Source: CAD feature listing. Evaluate the final solid. Frame: model axes, mm. A direction names the side the tool comes from. Give positions to 0.01 mm unless a question says otherwise; leave off trailing zeros. Loops run counter-clockwise (first coordinate to the right, second up) from the corner with the lowest first, then second, coordinate; pieces in that order, holes last. Notation, with made-up numbers: (-6, 77.25) - (1, 77.25) arc R26 cw to (1, 102.25) - close; hole circle Ø6 at (34.5, -2.75). An arc over 180 degrees is marked (long way). Put each result on its own line as item: value.
```python
from build123d import *

# Parameters (mm, degrees)
MODEL_R                 = 1.5
SALIENTE_EXTRUIR1_DEPTH = 3


with BuildPart() as part:
    # Model → Saliente-Extruir1 (new body)
    with BuildSketch(Plane.XY):
        with BuildLine():
            Line((256.429131311, 228.742243614), (346.429131311, 228.742243614))
            ThreePointArc((346.429131311, 228.742243614), (349.611111826, 227.424224129), (350.929131311, 224.242243614))
            Line((350.929131311, 224.242243614), (350.929131311, 215.242243614))
            ThreePointArc((350.929131311, 215.242243614), (349.611111826, 212.060263099), (346.429131311, 210.742243614))
            Line((346.429131311, 210.742243614), (256.429131311, 210.742243614))
            ThreePointArc((256.429131311, 210.742243614), (253.247150795, 212.060263099), (251.929131311, 215.242243614))
            Line((251.929131311, 215.242243614), (251.929131311, 224.242243614))
            ThreePointArc((251.929131311, 224.242243614), (253.247150795, 227.424224129), (256.429131311, 228.742243614))
        make_face()
        with Locations((337.429131311, 215.242243614)):
            Circle(MODEL_R, mode=Mode.SUBTRACT)
        with Locations((319.429131311, 215.242243614)):
            Circle(MODEL_R, mode=Mode.SUBTRACT)
        with Locations((328.429131311, 215.242243614)):
            Circle(MODEL_R, mode=Mode.SUBTRACT)
        with Locations((310.429131311, 215.242243614)):
            Circle(MODEL_R, mode=Mode.SUBTRACT)
        with Locations((292.429131311, 215.242243614)):
            Circle(MODEL_R, mode=Mode.SUBTRACT)
        with Locations((301.429131311, 215.242243614)):
            Circle(MODEL_R, mode=Mode.SUBTRACT)
        with Locations((274.429131311, 215.242243614)):
            Circle(MODEL_R, mode=Mode.SUBTRACT)
        with Locations((283.429131311, 215.242243614)):
            Circle(MODEL_R, mode=Mode.SUBTRACT)
        with Locations((265.429131311, 215.242243614)):
            Circle(MODEL_R, mode=Mode.SUBTRACT)
        with Locations((256.429131311, 215.242243614)):
            Circle(MODEL_R, mode=Mode.SUBTRACT)
        with Locations((346.429131311, 215.242243614)):
            Circle(MODEL_R, mode=Mode.SUBTRACT)
        with BuildLine():
            Line((256.429131311, 225.742243614), (346.429131311, 225.742243614))
            ThreePointArc((346.429131311, 225.742243614), (347.929131311, 224.242243614), (346.429131311, 222.742243614))
            Line((346.429131311, 222.742243614), (256.429131311, 222.742243614))
            ThreePointArc((256.429131311, 222.742243614), (254.929131311, 224.242243614), (256.429131311, 225.742243614))
        make_face(mode=Mode.SUBTRACT)
    extrude(amount=SALIENTE_EXTRUIR1_DEPTH)


solid = part.part
```
1) Section query A-A, the plane x = 297.5. Output: boundary loops of the cut face in (y, z).
Check result:
outline: (210.74, 0) - (222.74, 0) - (222.74, 3) - (210.74, 3) - close; (225.74, 0) - (228.74, 0) - (228.74, 3) - (225.74, 3) - close
2) Section query D-D, the plane y = 212.5. Output: boundary loops of the cut face in (x, z), plus the area to 3 significant figures.
Check result:
outline: (252.86, 0) - (350, 0) - (350, 3) - (252.86, 3) - close
area: 291 mm²
3) Material intervals for line 1 along Y through (x, z) = (301.5, 0.3); line 2 along Y through (x, z) = (282.5, 0.95); line 3 along Y through (x, z) = (278, 2.85), sorted ascending. Write a range as [from, to].
Check result:
line 1: [210.74, 213.74], [216.74, 222.74], [225.74, 228.74]
line 2: [210.74, 214.06], [216.42, 222.74], [225.74, 228.74]
line 3: [210.74, 222.74], [225.74, 228.74]
4) Mould query, pull axis Y, two halves, no side actions, for faces 1 (the flat face through (302, 220, 0)), 2 (the flat face through (301, 228.742, 1)), 3 (the cylindrical face through (300.324, 216.256, 1.479)). Classes: pulls with the +Y half, pulls with the -Y half, needs draft (parallel to the pull), parting line crosses it, or undercut.
Check result:
face 1: needs draft
face 2: pulls with the +Y half
face 3: undercut
5) Section query C-C, the plane x = 265.5. Output: boundary loops of the cut face in (y, z).
Check result:
outline: (210.74, 0) - (213.74, 0) - (213.74, 3) - (210.74, 3) - close; (216.74, 0) - (222.74, 0) - (222.74, 3) - (216.74, 3) - close; (225.74, 0) - (228.74, 0) - (228.74, 3) - (225.74, 3) - close
6) Access query for faces 4 (the flat face through (302, 210.742, 1)), 5 (the cylindrical face through (347.93, 224.28, 1.48)). Directions: +Z, -Z, +X, -X, +Y, -Y. A direction counts if a zero-diameter tool reaches every point of the face in a straight line with its end or side. Return the directions, or none.
Check result:
face 4: +Z, -Z, +X, -X, -Y
face 5: +Z, -Z
7) Pin query (flat end, axial travel): P1, Ø3.5, axis at x = 265.43, y = 215.24, coming from the -Z side; P2, Ø2.5, axis at x = 274.43, y = 215.24, coming from the -Z side. Return the tip coordinate at first contact, or that it passes through.
Check result:
P1: z = 0
P2: through
8) Section query B-B, the plane z = 1.85. State how many separate pieces and enclosed holes the cut face has, plus the area to 3 significant figures.
Check result:
separate pieces: 1
enclosed holes: 12
area: 1,410 mm²
